The model under review builds one solid part; all positions refer to its coordinate system, in mm. Face numbers are marked on the shaded views. A direction names the side the tool comes from. Coordinates: 2 decimals unless noted, no trailing zeros. Write each loop counter-clockwise with the first axis right and the second up, starting at its lowest first coordinate (ties: lowest second). Pieces come first, ordered by that corner, then holes. Notation, with made-up numbers: (71, -27) - (78, -27) arc R36 cw to (78, 12) - close; hole circle Ø10 at (84, 50.5). An arc over 180 degrees is marked (long way). Put each result on its own line as item: value. Start each with the question number.
Item 1: Machinability: for the marked faces 5 and 6, which of the approach directions +Z, -Z, +X, -X, +Y, -Y give a long, thin tool a straight path to every point of the face, cutting with its end or side? Answer none if there is none.
Item 2: Mouldability with a two-part tool opening along X and no side actions: class the marked faces 1, 2, 3 and 4 as pulls with the +X half, pulls with the -X half, needs draft (parallel to the pull), parting line crosses it, or undercut.
Item 3: Consider section D-D on x = -54. Give the boundary of the cut face in (y, z), then the cut area to 3 significant figures.
Item 4: Consider section B-B on y = -41.5. Give the boundary of the cut face in (x, z).
Item 5: Consider section C-C on z = 0.45. Give the boundary of the cut face in (x, y).
Item 6: For pin 1 (0.6 mm diameter, centred on x = -48, z = 3.5, fed in from -Y); pin 2 (0.8 mm diameter, centred on y = -29.5, z = 2.5, fed in from -X); pin 3 (0.8 mm diameter, centred on y = -32, z = 2, fed in from +X), all flat-tipped, find the tip position at first contact; note any pin that passes through.
Item 7: Consider section A-A on x = -50. Give the boundary of the cut face in (y, z).
Item 8: To check wall thickness, follow L1, parallel to X at y = -41.5, z = -0.25; L2, parallel to Y at x = -47.5, z = -0.35; L3, parallel to X at y = -42, z = 0.2 (3 decimals). State the ranges of each line that lie inside material, in increasing order. Write a range as [from, to].
```python
from build123d import *

# Parameters (mm, degrees)
SKETCH_1_W          = 33.9
SKETCH_1_H          = 34.2
SKETCH_1_W_2        = 27.9
SKETCH_1_H_2        = 28.2
EXTRUDE_1_DEPTH     = 4
SKETCH_2_W          = 33.9
SKETCH_2_H          = 34.2
EXTRUDE_2_DEPTH     = 2.2
FILLET_1_R          = 4
CUT_EXTRUDE_1_DEPTH = 0.6
FILLET_2_R          = 4
SKETCH_4_W          = 27.9
SKETCH_4_H          = 28.2
EXTRUDE_3_DEPTH     = 1.6
FILLET_3_R          = 1


with BuildPart() as part:
    # Эскиз1 → Бобышка-Вытянуть1 (new body)
    with BuildSketch(Plane.XY):
        with Locations((-48, -29.505896468)):
            Rectangle(SKETCH_1_W, SKETCH_1_H)
        with Locations((-48, -29.505896468)):
            Rectangle(SKETCH_1_W_2, SKETCH_1_H_2, mode=Mode.SUBTRACT)
    extrude(amount=EXTRUDE_1_DEPTH)

    # Эскиз2 → Бобышка-Вытянуть2 (add)
    with BuildSketch(Plane.XY.offset(4)):
        with Locations((-48, -29.505896468)):
            Rectangle(SKETCH_2_W, SKETCH_2_H)
        with BuildLine():
            Line((-60.85, -27.875896468), (-60.85, -33.635896468))
            ThreePointArc((-60.85, -33.635896468), (-59.385533906, -37.171430374), (-55.85, -38.635896468))
            Line((-55.85, -38.635896468), (-40.15, -38.635896468))
            ThreePointArc((-40.15, -38.635896468), (-36.614466094, -37.171430374), (-35.15, -33.635896468))
            Line((-35.15, -33.635896468), (-35.15, -27.875896468))
            ThreePointArc((-35.15, -27.875896468), (-36.614466094, -24.340362562), (-40.15, -22.875896468))
            Line((-40.15, -22.875896468), (-55.85, -22.875896468))
            ThreePointArc((-55.85, -22.875896468), (-59.385533906, -24.340362562), (-60.85, -27.875896468))
        make_face(mode=Mode.SUBTRACT)
    extrude(amount=-EXTRUDE_2_DEPTH)

    # Скругление1
    fillet_1_edges = [part.edges().sort_by_distance(p)[0] for p in [
        (-31.05, -46.605896468, 2),
        (-64.95, -46.605896468, 2),
        (-64.95, -12.405896468, 2),
        (-31.05, -12.405896468, 2),
    ]]
    fillet(fillet_1_edges, radius=FILLET_1_R)

    # Эскиз3 → Вырез-Вытянуть1 (cut)
    with BuildSketch(Plane.XY.offset(4)):
        with BuildLine():
            Line((-45, -19.640896468), (-51, -19.640896468))
            ThreePointArc((-51, -19.640896468), (-53, -17.640896468), (-51, -15.640896468))
            Line((-51, -15.640896468), (-45, -15.640896468))
            ThreePointArc((-45, -15.640896468), (-43, -17.640896468), (-45, -19.640896468))
        make_face()
    extrude(amount=-CUT_EXTRUDE_1_DEPTH, mode=Mode.SUBTRACT)

    # Скругление2
    # the kernel refuses this fillet: 4 mm, written as the material it takes off along each edge
    with BuildSketch(Plane(origin=(-35.05, -42.605896468, 4), x_dir=(0, -1, 0), z_dir=(-1, 0, 0))) as fillet_2_piece_1:
        with BuildLine():
            CenterArc((4 - FILLET_2_R, -FILLET_2_R), FILLET_2_R, 0, 90)
            Line((4, -FILLET_2_R), (4, 0))
            Line((4, 0), (4 - FILLET_2_R, 0))
        make_face()
    revolve(axis=Axis((-35.05, -42.605896468, 4), (0, 0, 1)), revolution_arc=90, mode=Mode.SUBTRACT)
    with BuildSketch(Plane(origin=(-60.95, -46.605896468, 4), x_dir=(0, 1, 0), z_dir=(1, 0, 0))) as fillet_2_piece_2:
        with BuildLine():
            CenterArc((FILLET_2_R, -FILLET_2_R), FILLET_2_R, 90, 90)
            Line((0, -FILLET_2_R), (0, 0))
            Line((0, 0), (FILLET_2_R, 0))
        make_face()
    extrude(amount=25.9, mode=Mode.SUBTRACT)
    with BuildSketch(Plane(origin=(-60.95, -42.605896468, 4), x_dir=(-1, 0, 0), z_dir=(0, 1, 0))) as fillet_2_piece_3:
        with BuildLine():
            CenterArc((4 - FILLET_2_R, -FILLET_2_R), FILLET_2_R, 0, 90)
            Line((4, -FILLET_2_R), (4, 0))
            Line((4, 0), (4 - FILLET_2_R, 0))
        make_face()
    revolve(axis=Axis((-60.95, -42.605896468, 4), (0, 0, 1)), revolution_arc=90, mode=Mode.SUBTRACT)
    with BuildSketch(Plane(origin=(-64.95, -16.405896468, 4), x_dir=(1, 0, 0), z_dir=(0, -1, 0)), Plane(origin=(-31.05, -42.605896468, 4), x_dir=(-1, 0, 0), z_dir=(0, 1, 0))) as fillet_2_piece_4:
        with BuildLine():
            CenterArc((FILLET_2_R, -FILLET_2_R), FILLET_2_R, 90, 90)
            Line((0, -FILLET_2_R), (0, 0))
            Line((0, 0), (FILLET_2_R, 0))
        make_face()
    extrude(amount=26.2, mode=Mode.SUBTRACT)
    with BuildSketch(Plane(origin=(-60.95, -16.405896468, 4), x_dir=(0, 1, 0), z_dir=(1, 0, 0))) as fillet_2_piece_5:
        with BuildLine():
            CenterArc((4 - FILLET_2_R, -FILLET_2_R), FILLET_2_R, 0, 90)
            Line((4 - FILLET_2_R, 0), (4, 0))
            Line((4, 0), (4, -FILLET_2_R))
        make_face()
    revolve(axis=Axis((-60.95, -16.405896468, 4), (0, 0, 1)), revolution_arc=90, mode=Mode.SUBTRACT)
    with BuildSketch(Plane(origin=(-35.05, -12.405896468, 4), x_dir=(0, 0, -1), z_dir=(-1, 0, 0))) as fillet_2_piece_6:
        with BuildLine():
            CenterArc((FILLET_2_R, FILLET_2_R), FILLET_2_R, 180, 90)
            Line((0, FILLET_2_R), (0, 0))
            Line((0, 0), (FILLET_2_R, 0))
        make_face()
    extrude(amount=25.9, mode=Mode.SUBTRACT)
    with BuildSketch(Plane(origin=(-35.05, -16.405896468, 4), x_dir=(0, 1, 0), z_dir=(-1, 0, 0))) as fillet_2_piece_7:
        with BuildLine():
            CenterArc((4 - FILLET_2_R, FILLET_2_R), FILLET_2_R, 270, 90)
            Line((4 - FILLET_2_R, 0), (4, 0))
            Line((4, 0), (4, FILLET_2_R))
        make_face()
    revolve(axis=Axis((-35.05, -16.405896468, 4), (0, 0, -1)), revolution_arc=90, mode=Mode.SUBTRACT)

    # Эскиз4 → Бобышка-Вытянуть3 (add)
    with BuildSketch(Plane(origin=(0, 0, 0), x_dir=(-1, 0, 0), z_dir=(0, 0, -1))):
        with BuildLine():
            Line((60.95, -12.405896468), (35.05, -12.405896468))
            ThreePointArc((35.05, -12.405896468), (32.221572875, -13.577469343), (31.05, -16.405896468))
            Line((31.05, -16.405896468), (31.05, -42.605896468))
            ThreePointArc((31.05, -42.605896468), (32.221572875, -45.434323593), (35.05, -46.605896468))
            Line((35.05, -46.605896468), (60.95, -46.605896468))
            ThreePointArc((60.95, -46.605896468), (63.778427125, -45.434323593), (64.95, -42.605896468))
            Line((64.95, -42.605896468), (64.95, -16.405896468))
            ThreePointArc((64.95, -16.405896468), (63.778427125, -13.577469343), (60.95, -12.405896468))
        make_face()
        with Locations((48, -29.505896468)):
            Rectangle(SKETCH_4_W, SKETCH_4_H, mode=Mode.SUBTRACT)
    extrude(amount=EXTRUDE_3_DEPTH)

    # Скругление3
    fillet_3_edges = [part.edges().sort_by_distance(p)[0] for p in [
        (-48, -38.635896468, 4),
        (-36.614466094, -37.171430374, 4),
        (-35.15, -30.755896468, 4),
        (-36.614466094, -24.340362562, 4),
        (-48, -22.875896468, 4),
        (-59.385533906, -24.340362562, 4),
        (-60.85, -30.755896468, 4),
        (-59.385533906, -37.171430374, 4),
    ]]
    fillet(fillet_3_edges, radius=FILLET_3_R)


solid = part.part
```
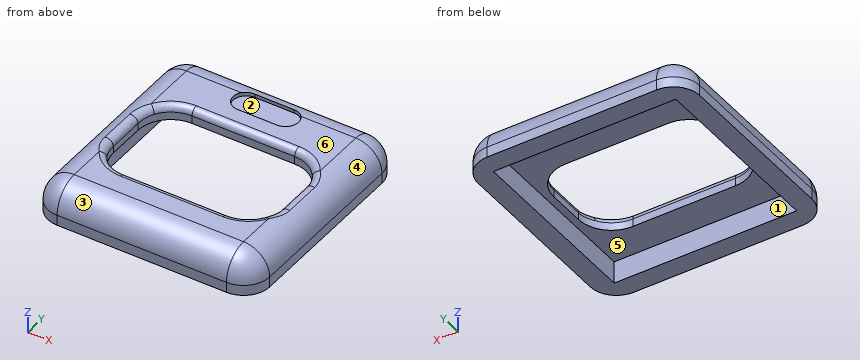
Report:
1. face 5: -Z
1. face 6: +Z, +X, -X, +Y, -Y
2. face 1: undercut
2. face 2: undercut
2. face 3: needs draft
2. face 4: pulls with the +X half
3. outline: (-46.61, -1.6) - (-43.61, -1.6) - (-43.61, 1.8) - (-38.64, 1.8) - (-38.64, 3) arc R1 ccw to (-39.64, 4) - (-42.61, 4) arc R4 ccw to (-46.61, 0) - close; (-22.88, 1.8) - (-15.41, 1.8) - (-15.41, -1.6) - (-12.41, -1.6) - (-12.41, 0) arc R4 ccw to (-16.41, 4) - (-21.88, 4) arc R1 ccw to (-22.88, 3) - close
3. area: 53.7 mm²
4. outline: (-64.95, -1.6) - (-61.95, -1.6) - (-61.95, 1.8) - (-34.05, 1.8) - (-34.05, -1.6) - (-31.05, -1.6) - (-31.05, 0) arc R4 ccw to (-35.05, 4) - (-60.95, 4) arc R4 ccw to (-64.95, 0) - close
5. outline: (-64.92, -42.61) arc R3.97 ccw to (-60.95, -46.58) - (-35.05, -46.58) arc R3.97 ccw to (-31.08, -42.61) - (-31.08, -16.41) arc R3.97 ccw to (-35.05, -12.43) - (-60.95, -12.43) arc R3.97 ccw to (-64.92, -16.41) - close; hole (-61.95, -43.61) - (-34.05, -43.61) - (-34.05, -15.41) - (-61.95, -15.41) - close
6. pin 1: y = -45.01
6. pin 2: x = -64.35
6. pin 3: x = -31.38
7. outline: (-46.61, -1.6) - (-43.61, -1.6) - (-43.61, 1.8) - (-38.64, 1.8) - (-38.64, 3) arc R1 ccw to (-39.64, 4) - (-42.61, 4) arc R4 ccw to (-46.61, 0) - close; (-22.88, 1.8) - (-15.41, 1.8) - (-15.41, -1.6) - (-12.41, -1.6) - (-12.41, 0) arc R4 ccw to (-15.64, 3.93) - (-15.64, 3.4) - (-19.64, 3.4) - (-19.64, 4) - (-21.88, 4) arc R1 ccw to (-22.88, 3) - close
8. L1: [-64.95, -61.95], [-34.05, -31.05]
8. L2: [-46.61, -43.61], [-15.41, -12.41]
8. L3: [-64.945, -61.95], [-34.05, -31.055]
